```python
from build123d import *

# Parameters (mm, degrees)
F0_W      = 1778
F0_H      = 1016
F1_DEPTH  = 1016
F2_W      = 762
F2_H      = 508
F3_DEPTH  = 508
F4_W      = 26.7618985716
F4_H      = 508
F5_DEPTH  = 508
F6_R      = 254
F7_R      = 254
F8_R      = 254
F9_DEPTH  = 508
F11_DEPTH = 254


with BuildPart() as f1:
    # F0 (on Top) → F1 (new body)
    with BuildSketch(Plane.XY):
        with Locations((133.4459019247, 5.0370320678)):
            Rectangle(F0_W, F0_H)
    extrude(amount=F1_DEPTH)

    # F2 (on face) → F3 (cut)
    with BuildSketch(Plane.XZ.offset(502.9629679322)):
        with Locations((-120.5540980753, 508)):
            Rectangle(F2_W, F2_H)
    extrude(amount=-F3_DEPTH, mode=Mode.SUBTRACT)

    # F4 (on face) → F5 (cut)
    with BuildSketch(Plane.XZ.offset(502.9629679322)):
        with Locations((247.0649526389, 508)):
            Rectangle(F4_W, F4_H)
        Polygon((1022.4459019247, 1016), (233.6840033531, 1016), (233.6840033531, 762), (260.4459019247, 762), (260.4459019247, 254), (233.6840033531, 254), (233.6840033531, 0), (1022.4459019247, 0), align=None)
    extrude(amount=-F5_DEPTH, mode=Mode.SUBTRACT)

    # F6
    f6_edges = [f1.edges().sort_by_distance(p)[0] for p in [
        (1022.445902, 259.037032, 1016),
    ]]
    fillet(f6_edges, radius=F6_R)

    # F7
    f7_edges = [f1.edges().sort_by_distance(p)[0] for p in [
        (1022.445902, 259.037032, 0),
    ]]
    fillet(f7_edges, radius=F7_R)

    # F8 (on face) → F9 (cut)
    with BuildSketch(Plane.XZ.offset(-5.0370320678)):
        with Locations((557.0327043533, 518.402338028)):
            Circle(F8_R)
    extrude(amount=-F9_DEPTH, mode=Mode.SUBTRACT)

    # F10 (on face) → F11 (cut)
    with BuildSketch(Plane(origin=(0, 0, 0), x_dir=(1, 0, 0), z_dir=(0, 0, -1))):
        Polygon((233.6840033531, -5.0370320678), (233.6840033531, 502.9629679322), (-274.3159966469, 502.9629679322), align=None)
    extrude(amount=-F11_DEPTH, mode=Mode.SUBTRACT)


solid = f1.part
```
Part model, mm, in its own coordinate system. A direction names the side the tool comes from. Round coordinates to 2 decimals unless told otherwise and drop trailing zeros. Loops run counter-clockwise (first coordinate to the right, second up) from the corner with the lowest first, then second, coordinate; pieces in that order, holes last. Notation, with made-up numbers: (-16.75, 38) -> (25.25, 38) arc R26 ccw to (25.25, 55) -> close; hole circle Ø5 at (14.5, -37). An arc over 180 degrees is marked (long way). Use CSV: the item, a comma, the result in double quotes. Start each with the question number.
1) Drop flat-ended pins along their axis: P1, Ø1.5, axis at x = 133, y = -234, coming from the -Z side; P2, Ø3, axis at y = -101.5, z = 783.5, coming from the +X side; P3, Ø6, axis at x = 734.5, z = 309, coming from the -Y side. Give the stop position or say it passes through.
2) Which spindle directions (+Z, -Z, +X, -X, +Y, -Y) get a long thin tool onto all of the face, cutting with end or side? Do faces 4 (the flat face through (-755.554, -2, 501)), 5 (the flat face through (-501.554, -253, 504)), 6 (the flat face through (-23.872, -252.519, 125.222)). Say none if no direction does.
3) Cut at C-C, the plane y = 361.5. Write the cut outline in (x, z).
4) Wall check: L1, parallel to Z at x = -482, y = -68.5; L2, parallel to X at y = -239.5, z = 344.5; L3, parallel to X at y = 192, z = 313. Give the ranges that are in metal, low to high. Write a range as [from, to].
5) Cut at B-B, the plane x = -439.5. Write the cut outline in (y, z), plus the area to 3 significant figures.
6) Pull direction Z, two halves, no side cores. Call faces 1 (the flat face through (250, 5.037, 515)), 2 (the flat face through (233.684, -253, 891)), 3 (the flat face through (-174, 12, 1016)): +Z half, -Z half, draft (parallel to the pull), parting line (faces both ways), or undercut.
7) Cut at A-A, the plane z = 656. Write the cut outline in (x, y), plus the area to 3 significant figures.
8) Cut at D-D, the plane x = 657.5. Write the cut outline in (y, z).
Determined:
1,P1,"stops at z = 762"
1,P2,"stops at x = 233.68"
1,P3,"stops at y = 5.04"
2,face 4,"+Z, -Z, -X, +Y, -Y"
2,face 5,"+X, -Y"
2,face 6,"-Z, +X, -Y"
3,outline,"(-755.55, 0) -> (768.45, 0) arc R254 ccw to (1022.45, 254) -> (1022.45, 762) arc R254 ccw to (768.45, 1016) -> (-755.55, 1016) -> close; hole circle Ø508 at (557.03, 518.4)"
4,L1,"z = [0, 254], [762, 1016]"
4,L2,"x = [-755.55, -501.55]"
4,L3,"x = [-755.55, 407.61], [706.45, 1022.45]"
5,outline,"(-502.96, 0) -> (513.04, 0) -> (513.04, 1016) -> (-502.96, 1016) -> (-502.96, 762) -> (5.04, 762) -> (5.04, 254) -> (-502.96, 254) -> close"
5,area,"774,000 mm2"
6,face 1,"undercut"
6,face 2,"draft"
6,face 3,"+Z half"
7,outline,"(-755.55, -502.96) -> (-501.55, -502.96) -> (-501.55, 5.04) -> (343.53, 5.04) -> (343.53, 513.04) -> (-755.55, 513.04) -> close; (770.53, 5.04) -> (1022.45, 5.04) -> (1022.45, 513.04) -> (770.53, 513.04) -> close"
7,area,"815,000 mm2"
8,outline,"(5.04, 0) -> (513.04, 0) -> (513.04, 285.12) -> (5.04, 285.12) -> close; (5.04, 751.69) -> (513.04, 751.69) -> (513.04, 1016) -> (5.04, 1016) -> close"
